The listing builds one solid part. Answer for the finished solid, in the listing's coordinates (mm). A direction names the side the tool comes from. Coordinates: 2 decimals unless noted, no trailing zeros. Write each loop counter-clockwise with the first axis right and the second up, starting at its lowest first coordinate (ties: lowest second). Pieces come first, ordered by that corner, then holes.
(1) Given P1, Ø3.5, axis at y = 0.5, z = -14.5, coming from the +X side; P2, Ø4, axis at y = -10, z = 45, coming from the -X side; P3, Ø1, axis at x = -0.5, z = 14.5, coming from the +Y side, each flat-ended and moving along its own axis, determine where each tip first touches the part or whether it passes through.
(2) Which of the six approach directions +Z, -Z, +X, -X, +Y, -Y give full straight-line access (tool end or side, diameter ignored) to faces 1 (the flat face through (0, 4.496, 1)), 2 (the flat face through (0, -3, 76.2)), 3 (the flat face through (5.55, -7.07, 1.07))?
(3) For a pull along Y with two mould halves and no side action, classify faces 4 (the flat face through (8, 12.7, 1)), 5 (the flat face through (7.066, 5.461, 1.067)), 6 (the flat face through (-12.7, -8, 1)) as +Y half, -Y half, draft (parallel to the pull), parting line (faces both ways), or undercut.
(4) Straight lines are drawn through the part: line 1 (Y direction, x = 0, z = -36); line 2 (Y direction, x = 6.25, z = 15); line 3 (Y direction, x = -7, z = 28). For each, find the intervals that lie inside material, in ascending order.
(5) The part is cut by section C-C on z = 51.5. Give the number of separate pieces and of enclosed holes in the cut face, plus the area to 3 significant figures.
(6) The part is cut by section A-A on x = 0. Determine the outline of the cut face in (y, z).
(7) The part is cut by section B-B on y = 0. Determine the outline of the cut face in (x, z), plus the area to 3 significant figures.
from build123d import *

# Parameters (mm, degrees)
SKETCH3_R                = 2.6035
BOSS_EXTRUDE1_DEPTH      = 76.2
BOSS_EXTRUDE1_DEPTH_BACK = 76.2


with BuildPart() as part:
    # Sketch3 → Boss-Extrude1 (new body, two sides)
    with BuildSketch(Plane.XY) as boss_extrude1_sk:
        with BuildLine():
            Line((6.3331344, -12.7), (9.5504, -12.7))
            ThreePointArc((9.5504, -12.7), (10.058323491, -12.192000006), (10.566399977, -12.699846982))
            ThreePointArc((10.566399977, -12.699846982), (12.082522516, -12.082522516), (12.699846982, -10.566399977))
            ThreePointArc((12.699846982, -10.566399977), (12.192000006, -10.058323491), (12.7, -9.5504))
            Line((12.7, -9.5504), (12.7, -6.3330836))
            ThreePointArc((12.7, -6.3330836), (12.192, -5.8250836), (12.7, -5.3170836))
            Line((12.7, -5.3170836), (12.7, -4.28752))
            ThreePointArc((12.7, -4.28752), (12.392749156, -3.545750844), (11.65098, -3.2385))
            Line((11.65098, -3.2385), (11.53922, -3.2385))
            ThreePointArc((11.53922, -3.2385), (10.797450844, -3.545750844), (10.4902, -4.28752))
            Line((10.4902, -4.28752), (10.4902, -6.402089023))
            ThreePointArc((10.4902, -6.402089023), (9.856394933, -7.351113629), (8.736962546, -7.129240479))
            Line((8.736962546, -7.129240479), (5.440484187, -3.838768792))
            ThreePointArc((5.440484187, -3.838768792), (4.75073678, -2.808015636), (4.5085, -1.591658411))
            Line((4.5085, -1.591658411), (4.5085, 1.591658411))
            ThreePointArc((4.5085, 1.591658411), (4.75073678, 2.808015636), (5.440484187, 3.838768792))
            Line((5.440484187, 3.838768792), (8.736962546, 7.129240479))
            ThreePointArc((8.736962546, 7.129240479), (9.856394933, 7.351113629), (10.4902, 6.402089023))
            Line((10.4902, 6.402089023), (10.4902, 4.28752))
            ThreePointArc((10.4902, 4.28752), (10.797450844, 3.545750844), (11.53922, 3.2385))
            Line((11.53922, 3.2385), (11.65098, 3.2385))
            ThreePointArc((11.65098, 3.2385), (12.392749156, 3.545750844), (12.7, 4.28752))
            Line((12.7, 4.28752), (12.7, 5.3171344))
            ThreePointArc((12.7, 5.3171344), (12.192, 5.8251344), (12.7, 6.3331344))
            Line((12.7, 6.3331344), (12.7, 9.5504))
            ThreePointArc((12.7, 9.5504), (12.192000006, 10.058323491), (12.699846982, 10.566399977))
            ThreePointArc((12.699846982, 10.566399977), (12.082522516, 12.082522516), (10.566399977, 12.699846982))
            ThreePointArc((10.566399977, 12.699846982), (10.058323491, 12.192000006), (9.5504, 12.7))
            Line((9.5504, 12.7), (6.3330836, 12.7))
            ThreePointArc((6.3330836, 12.7), (5.8250836, 12.192), (5.3170836, 12.7))
            Line((5.3170836, 12.7), (4.28752, 12.7))
            ThreePointArc((4.28752, 12.7), (3.545750844, 12.392749156), (3.2385, 11.65098))
            Line((3.2385, 11.65098), (3.2385, 11.53922))
            ThreePointArc((3.2385, 11.53922), (3.545750844, 10.797450844), (4.28752, 10.4902))
            Line((4.28752, 10.4902), (6.476795923, 10.4902))
            ThreePointArc((6.476795923, 10.4902), (7.432175542, 9.851520654), (7.207206853, 8.724555432))
            Line((7.207206853, 8.724555432), (3.900315394, 5.423689619))
            ThreePointArc((3.900315394, 5.423689619), (2.8709819, 4.736928798), (1.657299581, 4.4958))
            Line((1.657299581, 4.4958), (-1.553667902, 4.4958))
            ThreePointArc((-1.553667902, 4.4958), (-2.767350221, 4.736928798), (-3.796683715, 5.423689619))
            Line((-3.796683715, 5.423689619), (-7.134200223, 8.755124678))
            ThreePointArc((-7.134200223, 8.755124678), (-7.355273948, 9.862578342), (-6.416435163, 10.4902))
            Line((-6.416435163, 10.4902), (-4.28752, 10.4902))
            ThreePointArc((-4.28752, 10.4902), (-3.545750844, 10.797450844), (-3.2385, 11.53922))
            Line((-3.2385, 11.53922), (-3.2385, 11.65098))
            ThreePointArc((-3.2385, 11.65098), (-3.545750844, 12.392749156), (-4.28752, 12.7))
            Line((-4.28752, 12.7), (-5.3171344, 12.7))
            ThreePointArc((-5.3171344, 12.7), (-5.8251344, 12.192), (-6.3331344, 12.7))
            Line((-6.3331344, 12.7), (-9.5504, 12.7))
            ThreePointArc((-9.5504, 12.7), (-10.058323491, 12.192000006), (-10.566399977, 12.699846982))
            ThreePointArc((-10.566399977, 12.699846982), (-12.082522516, 12.082522516), (-12.699846982, 10.566399977))
            ThreePointArc((-12.699846982, 10.566399977), (-12.192000006, 10.058323491), (-12.7, 9.5504))
            Line((-12.7, 9.5504), (-12.7, 6.3331344))
            ThreePointArc((-12.7, 6.3331344), (-12.192, 5.8251344), (-12.7, 5.3171344))
            Line((-12.7, 5.3171344), (-12.7, -5.3170836))
            ThreePointArc((-12.7, -5.3170836), (-12.192, -5.8250836), (-12.7, -6.3330836))
            Line((-12.7, -6.3330836), (-12.7, -9.5504))
            ThreePointArc((-12.7, -9.5504), (-12.192000006, -10.058323491), (-12.699846982, -10.566399977))
            ThreePointArc((-12.699846982, -10.566399977), (-12.082522516, -12.082522516), (-10.566399977, -12.699846982))
            ThreePointArc((-10.566399977, -12.699846982), (-10.058323491, -12.192000006), (-9.5504, -12.7))
            Line((-9.5504, -12.7), (-6.3330836, -12.7))
            ThreePointArc((-6.3330836, -12.7), (-5.8250836, -12.192), (-5.3170836, -12.7))
            Line((-5.3170836, -12.7), (5.3171344, -12.7))
            ThreePointArc((5.3171344, -12.7), (5.8251344, -12.192), (6.3331344, -12.7))
        make_face()
        Circle(SKETCH3_R, mode=Mode.SUBTRACT)
        with BuildLine():
            Line((-8.753441447, -7.145689354), (-5.440484187, -3.838768792))
            ThreePointArc((-5.440484187, -3.838768792), (-4.75073678, -2.808015636), (-4.5085, -1.591658411))
            Line((-4.5085, -1.591658411), (-4.5085, 1.591658411))
            ThreePointArc((-4.5085, 1.591658411), (-4.75073678, 2.808015636), (-5.440484187, 3.838768792))
            Line((-5.440484187, 3.838768792), (-8.736962546, 7.129240479))
            ThreePointArc((-8.736962546, 7.129240479), (-9.856394933, 7.351113629), (-10.4902, 6.402089023))
            Line((-10.4902, 6.402089023), (-10.4902, -6.425372487))
            ThreePointArc((-10.4902, -6.425372487), (-9.862352148, -7.36547709), (-8.753441447, -7.145689354))
        make_face(mode=Mode.SUBTRACT)
        with BuildLine():
            Line((7.147805753, -8.66526257), (3.900315394, -5.423689619))
            ThreePointArc((3.900315394, -5.423689619), (2.8709819, -4.736928798), (1.657299581, -4.4958))
            Line((1.657299581, -4.4958), (-1.657299581, -4.4958))
            ThreePointArc((-1.657299581, -4.4958), (-2.8709819, -4.736928798), (-3.900315394, -5.423689619))
            Line((-3.900315394, -5.423689619), (-7.153722341, -8.671168377))
            ThreePointArc((-7.153722341, -8.671168377), (-7.374796065, -9.77862204), (-6.435957281, -10.406243698))
            Line((-6.435957281, -10.406243698), (6.427597582, -10.406243698))
            ThreePointArc((6.427597582, -10.406243698), (7.369631963, -9.776485757), (7.147805753, -8.66526257))
        make_face(mode=Mode.SUBTRACT)
    extrude(amount=BOSS_EXTRUDE1_DEPTH)
    extrude(boss_extrude1_sk.sketch, amount=-BOSS_EXTRUDE1_DEPTH_BACK)


solid = part.part
Model answer:
1. P1: stops at x = 4.58
1. P2: stops at x = -12.7
1. P3: stops at y = 4.5
2. face 1: +Z, -Z, +Y
2. face 2: +Z, +X, -X, +Y, -Y
2. face 3: +Z, -Z
3. face 4: +Y half
3. face 5: undercut
3. face 6: draft
4. line 1: y = -12.7 to -10.41, -4.5 to -2.6, 2.6 to 4.5
4. line 2: y = -12.42 to -10.41, -7.77 to -4.65, 4.65 to 7.77, 10.49 to 12.42
4. line 3: y = -12.7 to -10.24, -8.52 to -5.4, 5.4 to 8.62, 10.31 to 12.7
5. separate pieces: 1
5. enclosed holes: 3
5. area: 313 mm2
6. outline: (-12.7, -76.2) - (-10.41, -76.2) - (-10.41, 76.2) - (-12.7, 76.2) - close; (-4.5, -76.2) - (-2.6, -76.2) - (-2.6, 76.2) - (-4.5, 76.2) - close; (2.6, -76.2) - (4.5, -76.2) - (4.5, 76.2) - (2.6, 76.2) - close
7. outline: (-12.7, -76.2) - (-10.49, -76.2) - (-10.49, 76.2) - (-12.7, 76.2) - close; (-4.51, -76.2) - (-2.6, -76.2) - (-2.6, 76.2) - (-4.51, 76.2) - close; (2.6, -76.2) - (4.51, -76.2) - (4.51, 76.2) - (2.6, 76.2) - close
7. area: 917 mm2
